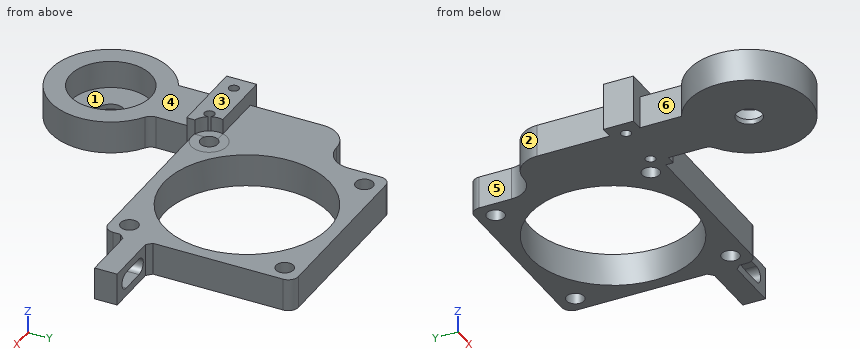
```python
from build123d import *
from build123d.topology import SkipClean

# Parameters (mm, degrees)
SKETCH1_R           = 8.05
SKETCH1_R_2         = 1.75
SKETCH1_R_3         = 12.5
BOSS_EXTRUDE3_DEPTH = 6.5
SKETCH1_5_R         = 2.55
BOSS_EXTRUDE2_DEPTH = 1
CUT_EXTRUDE1_DEPTH  = 10
FILLET2_R           = 2
FILLET5_R           = 5
CHAMFER2_SIZE       = 1
FILLET1_R           = 2
SKETCH5_R           = 16.5
CUT_EXTRUDE2_DEPTH  = 10
SKETCH4_R           = 1
CUT_EXTRUDE3_DEPTH  = 10
SKETCH4_4_W         = 1.918871126
SKETCH4_4_H         = 1.5
BOSS_EXTRUDE4_DEPTH = 6.5
SKETCH4_5_W         = 15.5
SKETCH4_5_H         = 6
BOSS_EXTRUDE5_DEPTH = 3
CUT_EXTRUDE5_START  = 9
SKETCH4_6_R         = 1
CUT_EXTRUDE5_DEPTH  = 9
SKETCH6_R           = 3.55
CUT_EXTRUDE6_DEPTH  = 8


with BuildPart() as part:
    # Sketch1 → Boss-Extrude3 (new body)
    with BuildSketch(Plane.XY):
        with BuildLine():
            ThreePointArc((-5.55, 10.695793566), (0, -12.05), (5.55, 10.695793566))
            Line((5.55, 10.695793566), (5.55, 20.5))
            Line((5.55, 20.5), (43, 20.5))
            Line((43, 20.5), (43, 25))
            Line((43, 25), (55, 25))
            Line((55, 25), (55, 29.5))
            Line((55, 29.5), (43, 29.5))
            Line((43, 29.5), (43, 58.5))
            Line((43, 58.5), (5, 58.5))
            Line((5, 58.5), (5, 45.05))
            Line((5, 45.05), (0, 45.05))
            ThreePointArc((0, 45.05), (-3.924442636, 43.424442636), (-5.55, 39.5))
            Line((-5.55, 39.5), (-5.55, 10.695793566))
        make_face()
        with Locations(Location((0, 0, 0), (0, 0, 180))):
            Circle(SKETCH1_R, mode=Mode.SUBTRACT)
        with Locations(Location((8.5, 24, 0), (0, 0, 180))):
            Circle(SKETCH1_R_2, mode=Mode.SUBTRACT)
        with Locations(Location((39.5, 24, 0), (0, 0, 180))):
            Circle(SKETCH1_R_2, mode=Mode.SUBTRACT)
        with Locations(Location((8.5, 55, 0), (0, 0, 180))):
            Circle(SKETCH1_R_2, mode=Mode.SUBTRACT)
        with Locations(Location((24, 39.5, 0), (0, 0, 180))):
            Circle(SKETCH1_R_3, mode=Mode.SUBTRACT)
        with Locations(Location((39.5, 55, 0), (0, 0, 180))):
            Circle(SKETCH1_R_2, mode=Mode.SUBTRACT)
    extrude(amount=BOSS_EXTRUDE3_DEPTH)

    # Sketch1<5> → Boss-Extrude2 (add)
    # profile 1 of 2: a face of its own
    with BuildSketch(Plane.XY):
        with BuildLine():
            Line((-5.55, 5.830951895), (-5.55, 0))
            ThreePointArc((-5.55, 0), (0, -5.55), (5.55, 0))
            Line((5.55, 0), (5.55, 5.830951895))
            ThreePointArc((5.55, 5.830951895), (0, 8.05), (-5.55, 5.830951895))
        make_face()
        Circle(SKETCH1_5_R, mode=Mode.SUBTRACT)
    # profile 2 of 2: a face of its own
    with BuildSketch(Plane.XY):
        with BuildLine():
            ThreePointArc((5.55, 0), (0, -5.55), (-5.55, 0))
            Line((-5.55, 0), (-5.55, 5.830951895))
            ThreePointArc((-5.55, 5.830951895), (-3.172144385, -7.398648525), (8.05, 0))
            ThreePointArc((8.05, 0), (7.398648525, 3.172144385), (5.55, 5.830951895))
            Line((5.55, 5.830951895), (5.55, 0))
        make_face()
    extrude(amount=BOSS_EXTRUDE2_DEPTH)

    # Sketch3 → Cut-Extrude1 (cut)
    with BuildSketch(Plane(origin=(0, 29.5, 0), x_dir=(1, 0, 0), z_dir=(0, 1, 0))):
        with BuildLine():
            Line((46.5, -1.6), (51.5, -1.6))
            ThreePointArc((51.5, -1.6), (53.15, -3.25), (51.5, -4.9))
            Line((51.5, -4.9), (46.5, -4.9))
            ThreePointArc((46.5, -4.9), (44.85, -3.25), (46.5, -1.6))
        make_face()
    extrude(amount=-CUT_EXTRUDE1_DEPTH, mode=Mode.SUBTRACT)

    # Fillet2
    fillet2_edges = [part.edges().sort_by_distance(p)[0] for p in [
        (5.55, 20.5, 3.25),
        (5.55, 10.695793566, 3.25),
    ]]
    fillet(fillet2_edges, radius=FILLET2_R)

    # Fillet5
    fillet5_edges = [part.edges().sort_by_distance(p)[0] for p in [
        (5, 45.05, 3.25),
    ]]
    fillet(fillet5_edges, radius=FILLET5_R - 0.0001)  # a hair under: the kernel refuses the full size

    # Chamfer2
    chamfer2_edges = [part.edges().sort_by_distance(p)[0] for p in [
        (43, 29.5, 3.25),
        (43, 25, 3.25),
    ]]
    chamfer(chamfer2_edges, length=CHAMFER2_SIZE)

    # Fillet1
    fillet1_edges = [part.edges().sort_by_distance(p)[0] for p in [
        (43, 20.5, 3.25),
        (5, 58.5, 3.25),
        (43, 58.5, 3.25),
    ]]
    fillet(fillet1_edges, radius=FILLET1_R)

    # Sketch5 → Cut-Extrude2 (cut)
    with BuildSketch(Plane.XY.offset(6.5)):
        with Locations((24, 39.5)):
            Circle(SKETCH5_R)
    extrude(amount=-CUT_EXTRUDE2_DEPTH, mode=Mode.SUBTRACT)

    # Sketch4 → Cut-Extrude3 (cut)
    with BuildSketch(Plane.XY.offset(6.5)):
        with Locations((4.468871126, 22)):
            Circle(SKETCH4_R)
        with Locations((-5.031128874, 22)):
            Circle(SKETCH4_R)
    extrude(amount=-CUT_EXTRUDE3_DEPTH, mode=Mode.SUBTRACT)

    # Sketch4<4> → Boss-Extrude4 (add)
    with BuildSketch(Plane.XY.offset(6.5)):
        with BuildLine():
            Line((-8.031128874, 25), (-8.031128874, 19))
            Line((-8.031128874, 19), (-5.55, 19))
            Line((-5.55, 19), (-5.55, 21.145147525))
            ThreePointArc((-5.55, 21.145147525), (-6.031128874, 22), (-5.55, 22.854852475))
            Line((-5.55, 22.854852475), (-5.55, 25))
            Line((-5.55, 25), (-8.031128874, 25))
        make_face()
        with Locations((6.509435563, 19.75)):
            Rectangle(SKETCH4_4_W, SKETCH4_4_H)
    extrude(amount=-BOSS_EXTRUDE4_DEPTH)

    # Sketch4<5> → Boss-Extrude5 (add)
    with BuildSketch(Plane.XY.offset(6.5)):
        with Locations((-0.281128874, 22)):
            Rectangle(SKETCH4_5_W, SKETCH4_5_H)
    extrude(amount=BOSS_EXTRUDE5_DEPTH)

    # Sketch4<6> → Cut-Extrude5 (cut)
    with SkipClean():  # the faces are left unmerged after this step: merging them gives an invalid solid
        with BuildSketch(Plane.XY.offset(6.5).offset(CUT_EXTRUDE5_START)):
            with Locations((4.468871126, 22)):
                Circle(SKETCH4_6_R)
            with Locations((-5.031128874, 22)):
                Circle(SKETCH4_6_R)
        extrude(amount=-CUT_EXTRUDE5_DEPTH, mode=Mode.SUBTRACT)
    add(part.part.scale(1), mode=Mode.REPLACE)  # the faces are merged on a copy

    # Sketch6 → Cut-Extrude6 (cut)
    with SkipClean():  # the faces are left unmerged after this step: merging them gives an invalid solid
        with BuildSketch(Plane.XY.offset(6.5)):
            with Locations((8.5, 24)):
                Circle(SKETCH6_R)
        extrude(amount=CUT_EXTRUDE6_DEPTH, mode=Mode.SUBTRACT)


solid = part.part
```
Geometry: final body of the model. Coordinates: model frame, mm. Face numbers are marked on the shaded views. A direction names the side the tool comes from. Round coordinates to 2 decimals unless told otherwise and drop trailing zeros. Loops run counter-clockwise (first coordinate to the right, second up) from the corner with the lowest first, then second, coordinate; pieces in that order, holes last. Notation, with made-up numbers: (23.25, 84) -> (72.25, 84) arc R16 cw to (72.25, 102) -> close; hole circle Ø7 at (11.25, -10). An arc over 180 degrees is marked (long way). Write each question's results on one line, items separated by ' | '.
Item 1: Pin query (flat end, axial travel): pin 1 Ø2 at (y, z) = (35, 3.5) entering from -X; pin 2 Ø5.5 at (x, y) = (39.5, 55) entering from +Z; pin 3 Ø5 at (y, z) = (53.5, 3.5) entering from -X. Return the tip coordinate at first contact, or that it passes through.
Answers below:
pin 1: stops at x = -5.55 | pin 2: stops at z = 6.5 | pin 3: stops at x = 5
Item 2: Cut plane B-B on z = 3.25. State how many separate pieces and enclosed holes the cut face has, and give its area (3 significant figures).
Answers below:
separate pieces: 2 | enclosed holes: 8 | area: 1,190 mm²
Item 3: Cut plane A-A on x = 24. Return the cut outline in (y, z).
Answers below:
outline: (20.5, 0) -> (23, 0) -> (23, 6.5) -> (20.5, 6.5) -> close; (56, 0) -> (58.5, 0) -> (58.5, 6.5) -> (56, 6.5) -> close
Item 4: Line query: probe 1 along Y at (x, z) = (0, 3.05); probe 2 along X at (y, z) = (22, 2.25); probe 3 along Y at (x, z) = (-8, 0.5). Output: solid intervals per line, ascending. Write a range as [from, to].
Answers below:
probe 1: y = [-12.05, -8.05], [8.05, 45.05] | probe 2: x = [-8.03, -6.03], [-4.03, 3.47], [5.47, 42.94] | probe 3: y = [-9.01, 9.01], [19, 25]
Item 5: Set-up query: the marked faces 4, 5 and 6. Return all of +Z, -Z, +X, -X, +Y, -Y with unobstructed straight access to the full face (end or side cutting, diameter ignored); none if empty.
Answers below:
face 4: +Z, +X, -X, -Y | face 5: +Z, -Z, -X, +Y | face 6: +Z, -Z, -X
Item 6: Cut plane D-D on y = 7. Return the cut outline in (x, z).
Answers below:
outline: (-9.81, 0) -> (9.81, 0) -> (9.81, 6.5) -> (3.98, 6.5) -> (3.98, 1) -> (-3.98, 1) -> (-3.98, 6.5) -> (-9.81, 6.5) -> close
Item 7: Cut plane C-C on y = 42. Return the cut outline in (x, z), and give its area (3 significant figures).
Answers below:
outline: (-4.96, 0) -> (7.69, 0) -> (7.69, 6.5) -> (-4.96, 6.5) -> close; (40.31, 0) -> (43, 0) -> (43, 6.5) -> (40.31, 6.5) -> close | area: 99.7 mm²
Item 8: Pull-direction query (Y, two-part tool) for the marked faces 1, 2 and 3; classes: pulls with the +Y half, pulls with the -Y half, needs draft (parallel to the pull), parting line crosses it, or undercut.
Answers below:
face 1: undercut | face 2: pulls with the +Y half | face 3: needs draft
